Design review of the part built by this model. Coordinates are the model's own, in mm. A direction names the side the tool comes from. Coordinates: 2 decimals unless noted, no trailing zeros. Order: outer loops, then holes, each group sorted by start corner. A loop starts at its lowest first (then second) coordinate and runs counter-clockwise, first axis right, second up.
Autodesk Inventor part; units mm, degrees
ref_plane "YZ Plane" through (0, 0, 0) normal (1, 0, 0) x (0, 1, 0)
ref_plane "XZ Plane" through (0, 0, 0) normal (0, 1, 0) x (-1, 0, 0)
ref_plane "XY Plane" through (0, 0, 0) normal (0, 0, 1) x (1, 0, 0)
sketch "Skizze1" plane through (0, 0, 0) normal (0, 1, 0) x (-1, 0, 0)
  line L0 (35, 2) -> (28, 2)
  line L1 (35, 2) -> (35, 0)
  line L2 (35, 0) -> (28, 0)
  line L3 (24.1541, 6.1963) -> (8, 7)
  line L4 (24.0547, 4.1988) -> (7.9503, 5)
  line L5 (31, 2) -> (31, 0) construction
  line L6 (8, 7) -> (0, 7)
  line L7 (0, 7) -> (0, 5)
  line L8 (0, 5) -> (7.9503, 5)
  arc A0 (27.0013, 3.05) -> (28, 2) centre (28, 3) ccw
  arc A1 (25.0038, 3.15) -> (28, 0) centre (28, 3) ccw
  arc A2 (25.0038, 3.15) -> (24.0547, 4.1988) centre (24.005, 3.2) ccw
  arc A3 (27.0013, 3.05) -> (24.1541, 6.1963) centre (24.005, 3.2) ccw
  point P0 (0, 0)
  dimension "d0" = 2
  dimension "d1" = 31
  dimension "d2" = 4
  dimension "d5" = 7
  dimension "d6" = 8
  dimension "d7" = 2
  dimension "d8" = 2
  dimension "d26" = 1
  dimension "d27" = 3
  dimension "d28" = 1
  dimension "d29" = 0.2
extrude "Extrusion1" add sketch "Skizze1" along normal mid plane 6
sketch "Skizze2" plane through (-35, 3, 2) normal (0, 0, 1) x (1, 0, 0)
  line L0 (0, 0) -> (7, 0)
  line L1 (0, -6) -> (0, 0)
  line L2 (7, -6) -> (0, -6)
  line L3 (7, -6) -> (7, 0)
  line L4 (35, -7.2) -> (35, 1.2)
  line L5 (-7, -3) -> (42, -3)
  point P0 (35, -3)
  point P1 (4, -3)
  dimension "d30" = 31
hole "Bohrung1" at (-31, 0, 2) direction (0, 0, -1) diameter 3.3 end through all
sketch "Skizze3" plane through (0, 3, 0) normal (0, 1, 0) x (1, 0, 0)
  line L0 (0, -5) -> (-7.9503, -5)
  line L1 (-0.0196, -5.3946) -> (-28.1986, -3.9926)
  line L2 (0, -5) -> (-4.1955, 0)
  line L3 (-4.1955, 0) -> (-5.762, 0)
  line L4 (-5.762, 0) -> (-1.5665, -5)
  line L5 (0, 1.4) -> (0, -8.4) construction
  point P0 (0, 0)
  point P1 (-28, 0)
  dimension "d19" = 40
  dimension "d20" = 1.2
extrude "Extrusion2" add sketch "Skizze3" against normal blind 4
pattern_linear "Rechteckige Anordnung1" count 2 spacing 6 along (-1, 0, 0) of "Extrusion2"
mirror "Spiegeln1" about plane through (0, 0, 0) normal (1, 0, 0) of "Extrusion1", "Bohrung1", "Extrusion2", "Rechteckige Anordnung1"
sketch "Skizze4" plane through (-8, -3, 7) normal (0, 0, 1) x (1, 0, 0)
  line L0 (8, 7.2) -> (8, -1.2) construction
  line L1 (0, 0) -> (16, 0) construction
  line L2 (-6, 0) -> (-4, 2)
  line L3 (-4, 2) -> (20, 2)
  line L4 (20, 2) -> (22, 0)
  line L5 (22, 0) -> (-6, 0)
  point P0 (8, 3)
  dimension "d31" = 2
  dimension "d32" = 24
  dimension "d33" = 45
extrude "Extrusion3" cut sketch "Skizze4" against normal through all
fillet "Rundung1" radius 2 4 edges at (-14, -3, 5.7002) (-12, -1, 5.7998) (12, -1, 5.7998) (14, -3, 5.7002)
properties part number "Dribbler Daempfer Oben" material "PVC, hart"
1. For faces 4 (the flat face through (-26, -3, 3)), 5 (the flat face through (-2.1, 1, 2.5)), 6 (the flat face through (9.63, 1.03, 2.54)), list the 3-axis set-ups (+Z, -Z, +X, -X, +Y, -Y) from which the entire face can be reached by the end or side of a thin tool; tool diameter is ignored.
2. Add section D-D (x = 3). Give the boundary of the cut face in (y, z).
3. Add section B-B (z = 1.25). Give the boundary of the cut face in (x, y), and give its area (3 significant figures).
4. Mouldability with a two-part tool opening along X and no side actions: class faces 1 (the flat face through (-35, 0, 1)), 2 (the flat face through (11, 1, 0)), 3 (the cylindrical face through (11.93, -1.15, 5.79)) as pulls with the +X half, pulls with the -X half, needs draft (parallel to the pull), parting line crosses it, or undercut.
5. Add section C-C (y = 0.05). State how many separate pieces and enclosed holes the cut face has, and give its area (3 significant figures).
6. To check wall thickness, follow line 1 (Y direction, x = -31, z = 1); line 2 (Y direction, x = 3, z = 6.5); line 3 (X direction, y = 2.05, z = 4). State the ranges of each line that lie inside material, in increasing order.
7. Add section A-A (x = 31). Give the boundary of the cut face in (y, z).
8. Insertion check: pin 1 (2 mm diameter, centred on x = 12.5, z = 2.5, fed in from +Y); pin 2 (1.5 mm diameter, centred on y = 2.5, z = 5, fed in from +X); pin 3 (3 mm diameter, centred on x = 12.5, y = -1, fed in from +Z); pin 4 (1.5 mm diameter, centred on y = -0.5, z = 4.5, fed in from +X). Each pin has a flat end and moves straight along its axis. Give the tip position at first contact, or say it passes through.
Solution:
1. face 4: +Z, -Z, +X, -X, -Y
1. face 5: -Z, +Y, -Y
1. face 6: +Y, -Y
2. outline: (-1, 1.42) - (3, 1.42) - (3, 3.29) - (-1, 3.29) - close; (-1, 5) - (3, 5) - (3, 7) - (-1, 7) - close
3. outline: (-35, -3) - (-25.56, -3) - (-25.56, 3) - (-35, 3) - close; (-10.71, -1) - (-9.15, -1) - (-9.15, 3) - (-10.71, 3) - close; (-4.71, -1) - (-3.15, -1) - (-3.15, 3) - (-4.71, 3) - close; (3.15, -1) - (4.71, -1) - (4.71, 3) - (3.15, 3) - close; (9.15, -1) - (10.71, -1) - (10.71, 3) - (9.15, 3) - close; (25.56, -3) - (35, -3) - (35, 3) - (25.56, 3) - close; hole circle Ø3.3 at (-31, 0); hole circle Ø3.3 at (31, 0)
3. area: 121 mm2
4. face 1: pulls with the -X half
4. face 2: needs draft
4. face 3: undercut
5. separate pieces: 3
5. enclosed holes: 0
5. area: 168 mm2
6. line 1: y = -3 to -1.65, 1.65 to 3
6. line 2: y = -1 to 3
6. line 3: x = -26.9 to -24.61, -8.41 to -6.84, -2.41 to -0.84, 0.84 to 2.41, 6.84 to 8.41, 24.61 to 26.9
7. outline: (-3, 0) - (-1.65, 0) - (-1.65, 2) - (-3, 2) - close; (1.65, 0) - (3, 0) - (3, 2) - (1.65, 2) - close
8. pin 1: passes through
8. pin 2: stops at x = 26.82
8. pin 3: stops at z = 6.85
8. pin 4: stops at x = 26.95
